Read the model definition and answer for the solid it produces. Units are mm, in the model's axes. A direction names the side the tool comes from. Coordinates: 2 decimals unless noted, no trailing zeros. Loops run counter-clockwise (first coordinate to the right, second up) from the corner with the lowest first, then second, coordinate; pieces in that order, holes last.
from build123d import *

# Parameters (mm, degrees)
F0_R     = 15.0004726412
F0_R_2   = 9.9068563463
F0_R_3   = 5.0694396424
F1_DEPTH = 9
F2_R     = 19.8859945384
F2_R_2   = 15.0004726412
F3_DEPTH = 3
F7_D     = 10
F8_D     = 20
F8_DEPTH = 12
F8_TIP   = 6.0086061903


with BuildPart() as f1:
    # F0 (on Front) → F1 (new body, symmetric)
    with BuildSketch(Plane.XZ):
        Circle(F0_R)
        Circle(F0_R_2, mode=Mode.SUBTRACT)
        Circle(F0_R_2)
        Circle(F0_R_3, mode=Mode.SUBTRACT)
        Circle(F0_R_3)
    extrude(amount=F1_DEPTH, both=True)

    # F2 (on face) → F3 (join)
    with BuildSketch(Plane.XZ.offset(9)):
        Circle(F2_R)
        Circle(F2_R_2, mode=Mode.SUBTRACT)
    extrude(amount=-F3_DEPTH)

    # F4: F1 across plane


with BuildPart() as f1_1:
    add(f1.part)
    add(f1.part.mirror(Plane.XZ))

    # F5 (on Right) → F6 (revolve)
    with BuildSketch(Plane.YZ):
        Polygon((-3.5, 14.9199490446), (-5.9903608635, 19.839907065), (-5.9903608635, 14.9199490446), align=None)
        Polygon((5.9543419629, 14.9199490446), (5.9903608635, 19.839907065), (3.5, 14.9199490446), align=None)
    revolve(axis=Axis((0, 0, 0), (0, -1, 0)))

    # F7 (through all)
    with Locations(Plane.XZ.offset(9)):
        with Locations((0, 0)):
            Hole(F7_D / 2)

    # F8
    with Locations(Plane.XZ.offset(9)):
        with Locations((0, 0)):
            Hole(F8_D / 2, depth=F8_DEPTH)
            with Locations((0, 0, -(F8_DEPTH + F8_TIP / 2))):  # 118° drill point
                Cone(0, F8_D / 2, F8_TIP, mode=Mode.SUBTRACT)


solid = f1_1.part
Q1. Determine the mould class of faces 1 (the face through (-5, -9, 9)), 2 (the face through (13.52, 3.66, 7.03)), 3 (the face through (2.17, -2.92, -9.76)) for opening direction X: +X half, -X half, draft (parallel to the pull), parting line (faces both ways), or undercut.
Findings below:
face 1: draft
face 2: parting line
face 3: undercut
Q2. Which of the six approach directions +Z, -Z, +X, -X, +Y, -Y give full straight-line access (tool end or side, diameter ignored) to faces 4 (the face through (-4.311, -7.521, -19.413)), 5 (the face through (14.308, -0.05, 4.506))?
Findings below:
face 4: +Y, -Y
face 5: none
Q3. Straight lines are drawn through the part: probe 1 along X at (y, z) = (1.5, 0); probe 2 along Z at (x, y) = (2, -0.25). For each, find the intervals that lie inside material, in ascending order.
Findings below:
probe 1: x = -15 to -10, 10 to 15
probe 2: z = -14.87 to -9.8, 9.8 to 14.87
Q4. A cutting plane is placed at D-D (y = 6.5). Give the vertices of the cut face in (x, z).
Findings below:
outline: circle Ø39.77 at (0, 0); hole circle Ø10 at (0, 0)
Q5. Flat-ended cylindrical pins translate along their axes: pin 1 Ø6 at (x, y) = (12.5, 0.5) entering from +Z; pin 2 Ø20 at (x, z) = (2, 8.5) entering from -Y; pin 3 Ø4 at (x, y) = (-13, 0.5) entering from -Z; pin 4 Ø1.5 at (x, z) = (6.5, -3.5) entering from -Y. Find the tip coordinate at first contact, or state that the pin passes through.
Findings below:
pin 1: stops at z = 11.61
pin 2: stops at y = -9
pin 3: stops at z = -10.2
pin 4: stops at y = 4.12
Q6. A cutting plane is placed at C-C (y = -2). Give the vertices of the cut face in (x, z), then the cut area to 3 significant figures.
Findings below:
outline: circle Ø30 at (0, 0); hole circle Ø20 at (0, 0)
area: 393 mm2
